Verification items for the finished model (mm, model axes). Give positions to 0.01 mm unless a question says otherwise; leave off trailing zeros. Loops run counter-clockwise (first coordinate to the right, second up) from the corner with the lowest first, then second, coordinate; pieces in that order, holes last. Notation, with made-up numbers: (16, -10.5) - (48, -10.5) arc R19 cw to (48, -6.5) - close; hole circle Ø1 at (-31.5, 6.25). An arc over 180 degrees is marked (long way). Use one line per item in the form item = value.
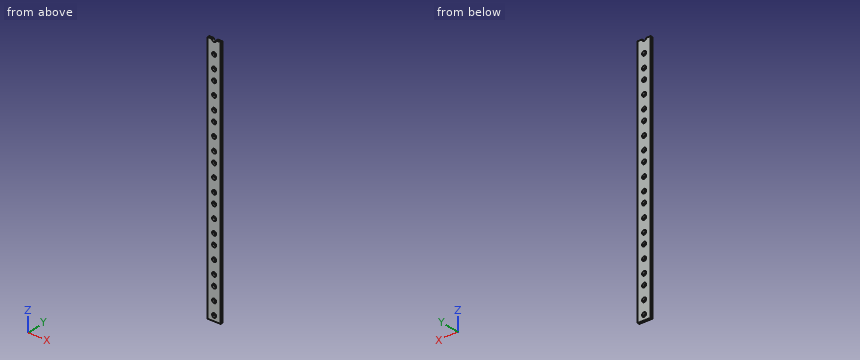
```python
from build123d import *

# Parameters (mm, degrees)
SKETCH1_W                  = 15.875
SKETCH1_H                  = 304.8
BOSS_EXTRUDE1_DEPTH        = 2.54
SKETCH2_R                  = 2.5527
CUT_EXTRUDE1_DEPTH         = 2.54
LPATTERN1_COUNT            = 3
LPATTERN1_PITCH            = 15.875
LPATTERN2_COUNT            = 7
LPATTERN2_PITCH            = 44.45
LPATTERN2_COPY_1_SKETCH_R  = 2.5527
LPATTERN2_COPY_1_DEPTH     = 2.54
LPATTERN2_COPY_2_SKETCH_R  = 2.5527
LPATTERN2_COPY_2_DEPTH     = 2.54
LPATTERN2_COPY_3_SKETCH_R  = 2.5527
LPATTERN2_COPY_3_DEPTH     = 2.54
LPATTERN2_COPY_4_SKETCH_R  = 2.5527
LPATTERN2_COPY_4_DEPTH     = 2.54
LPATTERN2_COPY_5_SKETCH_R  = 2.5527
LPATTERN2_COPY_5_DEPTH     = 2.54
LPATTERN2_COPY_6_SKETCH_R  = 2.5527
LPATTERN2_COPY_6_DEPTH     = 2.54
LPATTERN2_COPY_7_SKETCH_R  = 2.5527
LPATTERN2_COPY_7_DEPTH     = 2.54
LPATTERN2_COPY_8_SKETCH_R  = 2.5527
LPATTERN2_COPY_8_DEPTH     = 2.54
LPATTERN2_COPY_9_SKETCH_R  = 2.5527
LPATTERN2_COPY_9_DEPTH     = 2.54
LPATTERN2_COPY_10_SKETCH_R = 2.5527
LPATTERN2_COPY_10_DEPTH    = 2.54
LPATTERN2_COPY_11_SKETCH_R = 2.5527
LPATTERN2_COPY_11_DEPTH    = 2.54
LPATTERN2_COPY_12_SKETCH_R = 2.5527
LPATTERN2_COPY_12_DEPTH    = 2.54


with BuildPart() as part:
    # Sketch1 → Boss-Extrude1 (new body)
    with BuildSketch(Plane(origin=(0, 0, 0), x_dir=(1, 0, 0), z_dir=(0, 1, 0))):
        Rectangle(SKETCH1_W, SKETCH1_H)
    extrude(amount=BOSS_EXTRUDE1_DEPTH)

    # Sketch2 → Cut-Extrude1 (cut)
    with BuildSketch(Plane(origin=(0, 2.54, 0), x_dir=(1, 0, 0), z_dir=(0, 1, 0))):
        with Locations(Location((0, 146.05, 0), (0, 0, 270))):
            Circle(SKETCH2_R)
    cut_extrude1 = extrude(amount=-CUT_EXTRUDE1_DEPTH, mode=Mode.SUBTRACT)

    # LPattern1: Cut-Extrude1 ×3
    with Locations(*[(0, 0, i * LPATTERN1_PITCH) for i in range(1, LPATTERN1_COUNT)]):
        add(cut_extrude1, mode=Mode.SUBTRACT)

    # LPattern2: Cut-Extrude1 ×7
    with Locations(*[(0, 0, i * LPATTERN2_PITCH) for i in range(1, LPATTERN2_COUNT)]):
        add(cut_extrude1, mode=Mode.SUBTRACT)

    # LPattern2 copy 1 sketch → LPattern2 copy 1 (cut)
    with BuildSketch(Plane(origin=(0, 2.54, 60.325), x_dir=(1, 0, 0), z_dir=(0, 1, 0))):
        with Locations(Location((0, 146.05, 0), (0, 0, 270))):
            Circle(LPATTERN2_COPY_1_SKETCH_R)
    extrude(amount=-LPATTERN2_COPY_1_DEPTH, mode=Mode.SUBTRACT)

    # LPattern2 copy 2 sketch → LPattern2 copy 2 (cut)
    with BuildSketch(Plane(origin=(0, 2.54, 104.775), x_dir=(1, 0, 0), z_dir=(0, 1, 0))):
        with Locations(Location((0, 146.05, 0), (0, 0, 270))):
            Circle(LPATTERN2_COPY_2_SKETCH_R)
    extrude(amount=-LPATTERN2_COPY_2_DEPTH, mode=Mode.SUBTRACT)

    # LPattern2 copy 3 sketch → LPattern2 copy 3 (cut)
    with BuildSketch(Plane(origin=(0, 2.54, 149.225), x_dir=(1, 0, 0), z_dir=(0, 1, 0))):
        with Locations(Location((0, 146.05, 0), (0, 0, 270))):
            Circle(LPATTERN2_COPY_3_SKETCH_R)
    extrude(amount=-LPATTERN2_COPY_3_DEPTH, mode=Mode.SUBTRACT)

    # LPattern2 copy 4 sketch → LPattern2 copy 4 (cut)
    with BuildSketch(Plane(origin=(0, 2.54, 193.675), x_dir=(1, 0, 0), z_dir=(0, 1, 0))):
        with Locations(Location((0, 146.05, 0), (0, 0, 270))):
            Circle(LPATTERN2_COPY_4_SKETCH_R)
    extrude(amount=-LPATTERN2_COPY_4_DEPTH, mode=Mode.SUBTRACT)

    # LPattern2 copy 5 sketch → LPattern2 copy 5 (cut)
    with BuildSketch(Plane(origin=(0, 2.54, 238.125), x_dir=(1, 0, 0), z_dir=(0, 1, 0))):
        with Locations(Location((0, 146.05, 0), (0, 0, 270))):
            Circle(LPATTERN2_COPY_5_SKETCH_R)
    extrude(amount=-LPATTERN2_COPY_5_DEPTH, mode=Mode.SUBTRACT)

    # LPattern2 copy 6 sketch → LPattern2 copy 6 (cut)
    with BuildSketch(Plane(origin=(0, 2.54, 282.575), x_dir=(1, 0, 0), z_dir=(0, 1, 0))):
        with Locations(Location((0, 146.05, 0), (0, 0, 270))):
            Circle(LPATTERN2_COPY_6_SKETCH_R)
    extrude(amount=-LPATTERN2_COPY_6_DEPTH, mode=Mode.SUBTRACT)

    # LPattern2 copy 7 sketch → LPattern2 copy 7 (cut)
    with BuildSketch(Plane(origin=(0, 2.54, 76.2), x_dir=(1, 0, 0), z_dir=(0, 1, 0))):
        with Locations(Location((0, 146.05, 0), (0, 0, 270))):
            Circle(LPATTERN2_COPY_7_SKETCH_R)
    extrude(amount=-LPATTERN2_COPY_7_DEPTH, mode=Mode.SUBTRACT)

    # LPattern2 copy 8 sketch → LPattern2 copy 8 (cut)
    with BuildSketch(Plane(origin=(0, 2.54, 120.65), x_dir=(1, 0, 0), z_dir=(0, 1, 0))):
        with Locations(Location((0, 146.05, 0), (0, 0, 270))):
            Circle(LPATTERN2_COPY_8_SKETCH_R)
    extrude(amount=-LPATTERN2_COPY_8_DEPTH, mode=Mode.SUBTRACT)

    # LPattern2 copy 9 sketch → LPattern2 copy 9 (cut)
    with BuildSketch(Plane(origin=(0, 2.54, 165.1), x_dir=(1, 0, 0), z_dir=(0, 1, 0))):
        with Locations(Location((0, 146.05, 0), (0, 0, 270))):
            Circle(LPATTERN2_COPY_9_SKETCH_R)
    extrude(amount=-LPATTERN2_COPY_9_DEPTH, mode=Mode.SUBTRACT)

    # LPattern2 copy 10 sketch → LPattern2 copy 10 (cut)
    with BuildSketch(Plane(origin=(0, 2.54, 209.55), x_dir=(1, 0, 0), z_dir=(0, 1, 0))):
        with Locations(Location((0, 146.05, 0), (0, 0, 270))):
            Circle(LPATTERN2_COPY_10_SKETCH_R)
    extrude(amount=-LPATTERN2_COPY_10_DEPTH, mode=Mode.SUBTRACT)

    # LPattern2 copy 11 sketch → LPattern2 copy 11 (cut)
    with BuildSketch(Plane(origin=(0, 2.54, 254), x_dir=(1, 0, 0), z_dir=(0, 1, 0))):
        with Locations(Location((0, 146.05, 0), (0, 0, 270))):
            Circle(LPATTERN2_COPY_11_SKETCH_R)
    extrude(amount=-LPATTERN2_COPY_11_DEPTH, mode=Mode.SUBTRACT)

    # LPattern2 copy 12 sketch → LPattern2 copy 12 (cut)
    with BuildSketch(Plane(origin=(0, 2.54, 298.45), x_dir=(1, 0, 0), z_dir=(0, 1, 0))):
        with Locations(Location((0, 146.05, 0), (0, 0, 270))):
            Circle(LPATTERN2_COPY_12_SKETCH_R)
    extrude(amount=-LPATTERN2_COPY_12_DEPTH, mode=Mode.SUBTRACT)


solid = part.part
```
1. Scan lines: probe 1 along X at (y, z) = (2, 31.75); probe 2 along X at (y, z) = (1.8, 49). Record each from-to range of solid material in increasing order.
Result set:
probe_1 = -7.94 to -2.55, 2.55 to 7.94
probe_2 = -7.94 to -2.15, 2.15 to 7.94
2. Section check B-B, the plane y = 2.1. State how many separate pieces and enclosed holes the cut face has, then the cut area to 3 significant figures.
Result set:
separate_pieces = 1
enclosed_holes = 20
area = 4,420 mm²
3. Section check A-A, the plane z = 63.5. Record the cut outline in (x, y), then the cut area to 3 significant figures.
Result set:
outline = (-7.94, 0) - (-2.55, 0) - (-2.55, 2.54) - (-7.94, 2.54) - close; (2.55, 0) - (7.94, 0) - (7.94, 2.54) - (2.55, 2.54) - close
area = 27.4 mm²
